```python
from build123d import *

# Parameters (mm, degrees)
SKETCH1_W                       = 90
SKETCH1_H                       = 40
BOSS_EXTRUDE1_DEPTH             = 20
SKETCH2_W                       = 20
SKETCH2_H                       = 10
CUT_EXTRUDE1_DEPTH              = 54.150729064
SKETCH3_W                       = 20
SKETCH3_H                       = 10
CUT_EXTRUDE2_DEPTH              = 54.150729064
SKETCH4_W                       = 20
SKETCH4_H                       = 10
CUT_EXTRUDE3_DEPTH              = 54.150729064
SKETCH5_W                       = 20
SKETCH5_H                       = 10
CUT_EXTRUDE4_DEPTH              = 54.150729064
F_5_0_5_DIAMETER_HOLE1_D        = 5
F_5_0_5_DIAMETER_HOLE1_DEPTH    = 12
M27_CLEARANCE_HOLE1_D           = 29.849192884
F_10_0_10_DIAMETER_HOLE1_REACH  = 63.033
F_10_0_10_DIAMETER_HOLE1_BORE_R = 5
F_12_0_12_DIAMETER_HOLE1_D      = 12
CHAMFER1_SIZE                   = 2
SKETCH18_R                      = 6.25
CUT_EXTRUDE6_DEPTH              = 100
SKETCH20_R                      = 15.175
CUT_EXTRUDE7_DEPTH              = 100
SKETCH21_R                      = 2.75
CUT_EXTRUDE8_DEPTH              = 12
SKETCH23_R                      = 5
BOSS_EXTRUDE2_DEPTH             = 20


with BuildPart() as part:
    # Sketch1 → Boss-Extrude1 (new body)
    with BuildSketch(Plane.XY.offset(10)):
        Rectangle(SKETCH1_W, SKETCH1_H)
    extrude(amount=-BOSS_EXTRUDE1_DEPTH)

    # Sketch2 → Cut-Extrude1 (cut, through all)
    with BuildSketch(Plane(origin=(0, 0, -10), x_dir=(-1, 0, 0), z_dir=(0, 0, -1))):
        with Locations((35, 15)):
            Rectangle(SKETCH2_W, SKETCH2_H)
    extrude(amount=-CUT_EXTRUDE1_DEPTH, mode=Mode.SUBTRACT)

    # Sketch3 → Cut-Extrude2 (cut, through all)
    with BuildSketch(Plane(origin=(0, 0, -10), x_dir=(-1, 0, 0), z_dir=(0, 0, -1))):
        with Locations((35, -15)):
            Rectangle(SKETCH3_W, SKETCH3_H)
    extrude(amount=-CUT_EXTRUDE2_DEPTH, mode=Mode.SUBTRACT)

    # Sketch4 → Cut-Extrude3 (cut, through all)
    with BuildSketch(Plane(origin=(0, 0, -10), x_dir=(-1, 0, 0), z_dir=(0, 0, -1))):
        with Locations((-35, -15)):
            Rectangle(SKETCH4_W, SKETCH4_H)
    extrude(amount=-CUT_EXTRUDE3_DEPTH, mode=Mode.SUBTRACT)

    # Sketch5 → Cut-Extrude4 (cut, through all)
    with BuildSketch(Plane(origin=(0, 0, -10), x_dir=(-1, 0, 0), z_dir=(0, 0, -1))):
        with Locations((-35, 15)):
            Rectangle(SKETCH5_W, SKETCH5_H)
    extrude(amount=-CUT_EXTRUDE4_DEPTH, mode=Mode.SUBTRACT)

    # Ø5.0 (5) Diameter Hole1
    with Locations(Plane.XY.offset(10)):
        with Locations((20, 0), (-20, 0)):
            Hole(F_5_0_5_DIAMETER_HOLE1_D / 2, depth=F_5_0_5_DIAMETER_HOLE1_DEPTH)

    # M27 Clearance Hole1 (through all)
    with Locations(Plane.XY.offset(10)):
        with Locations((0, 0)):
            Hole(M27_CLEARANCE_HOLE1_D / 2)

    # Ø10.0 (10) Diameter Hole1 bore → Ø10.0 (10) Diameter Hole1 (cut, up to next)
    with BuildSketch(Plane(origin=(0, -20, 0), x_dir=(-1, 0, 0), z_dir=(0, -1, 0)), mode=Mode.PRIVATE) as f_10_0_10_diameter_hole1_sk1:
        Circle(F_10_0_10_DIAMETER_HOLE1_BORE_R)
    f_10_0_10_diameter_hole1_tool1 = extrude(f_10_0_10_diameter_hole1_sk1.sketch, amount=-F_10_0_10_DIAMETER_HOLE1_REACH, mode=Mode.PRIVATE) & part.part
    add(f_10_0_10_diameter_hole1_tool1.solids().sort_by_distance((0, -20, 0))[0], mode=Mode.SUBTRACT)

    # Ø12.0 (12) Diameter Hole1 (through all)
    with Locations(Plane(origin=(0, 0, -10), x_dir=(-1, 0, 0), z_dir=(0, 0, -1))):
        with Locations((35, 0), (-35, 0)):
            Hole(F_12_0_12_DIAMETER_HOLE1_D / 2)

    # Chamfer1
    chamfer1_edges = [part.edges().sort_by_distance(p)[0] for p in [
        (-25, 20, 0),
        (-45, 10, 0),
        (-45, -10, 0),
        (-25, -20, 0),
        (25, -20, 0),
        (45, -10, 0),
        (45, 10, 0),
        (25, 20, 0),
    ]]
    chamfer(chamfer1_edges, length=CHAMFER1_SIZE)

    # Sketch18 → Cut-Extrude6 (cut)
    with BuildSketch(Plane.XY.offset(10)):
        with Locations((-35, 0)):
            Circle(SKETCH18_R)
        with Locations((35, 0)):
            Circle(SKETCH18_R)
    extrude(amount=-CUT_EXTRUDE6_DEPTH, mode=Mode.SUBTRACT)

    # Sketch20 → Cut-Extrude7 (cut)
    with BuildSketch(Plane.XY.offset(10)):
        Circle(SKETCH20_R)
    extrude(amount=-CUT_EXTRUDE7_DEPTH, mode=Mode.SUBTRACT)

    # Sketch21 → Cut-Extrude8 (cut)
    with BuildSketch(Plane.XY.offset(10)):
        with Locations((-20, 0)):
            Circle(SKETCH21_R)
        with Locations(Location((20, 0, 0), (0, 0, 180))):
            Circle(SKETCH21_R)
    extrude(amount=-CUT_EXTRUDE8_DEPTH, mode=Mode.SUBTRACT)

    # Sketch23 → Boss-Extrude2 (add)
    with BuildSketch(Plane.XZ.offset(10)):
        with Locations(Location((-33.846356211, 0, 0), (0, 0, 90))):
            Circle(SKETCH23_R)
        with Locations(Location((33.846356211, 0, 0), (0, 0, 90))):
            Circle(SKETCH23_R)
    extrude(amount=BOSS_EXTRUDE2_DEPTH)


solid = part.part
```
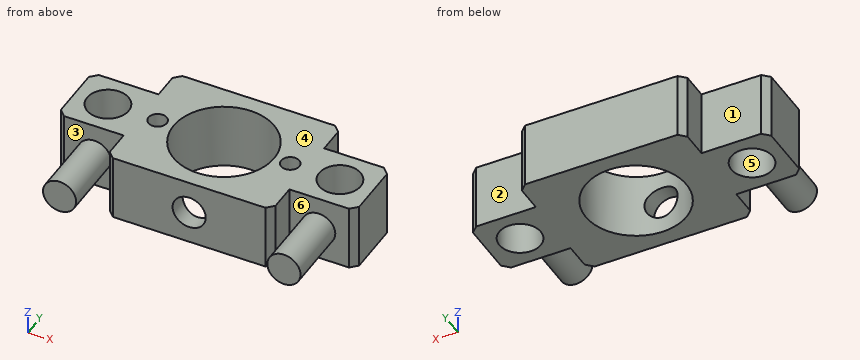
Verification items for the finished model (mm, model axes). Face numbers are marked on the shaded views. A direction names the side the tool comes from. Round coordinates to 2 decimals unless told otherwise and drop trailing zeros. Write each loop counter-clockwise with the first axis right and the second up, starting at its lowest first coordinate (ties: lowest second). Pieces come first, ordered by that corner, then holes.
1. Scan lines: L1, parallel to X at y = -16.55, z = 0; L2, parallel to X at y = -1, z = -1; L3, parallel to X at y = -16, z = -3.75. Record each from-to range of solid material in increasing order.
2. Section check B-B on x = 35. Enter the section's corners in (y, z), plus the area to 3 significant figures.
3. Access from +Z, -Z, +X, -X, +Y, -Y to the whole of each face (thin tool, end or side, straight path). Record for the marked faces 1, 2 and 3.
4. Draft check along Y on the marked faces 4, 5 and 6. Enter one of: +Y half, -Y half, draft (parallel to the pull), parting line (faces both ways), or undercut.
5. Section check D-D on z = 0. State how many separate pieces and enclosed holes the cut face has, plus the area to 3 significant figures.
6. Section check A-A on y = 0. Enter the section's corners in (x, z) (3 decimals).
7. Section check C-C on x = -2. Enter the section's corners in (y, z), plus the area to 3 significant figures.
8. Gauge pin test, flat ends, axial feed: P1, Ø2.5, axis at y = 12.5, z = 1, coming from the -X side; P2, Ø1.6, axis at x = 21, y = 1, coming from the +Z side; P3, Ø10, axis at x = -14.5, z = -4.5, coming from the -Y side. Record the tip position at first contact, or that the pin passes through.
Answer:
1. L1: x = -38.85 to -28.85, -25 to -5, 5 to 25, 28.85 to 38.85
1. L2: x = -45 to -41.17, -28.83 to -22.56, -17.44 to -15.14, 15.14 to 17.44, 22.56 to 28.83, 41.17 to 45
1. L3: x = -37.15 to -30.54, -25 to -3.31, 3.31 to 25, 30.54 to 37.15
2. outline: (-30, -4.87) - (-10, -4.87) - (-10, -10) - (-6.25, -10) - (-6.25, 10) - (-10, 10) - (-10, 4.87) - (-30, 4.87) - close; (6.25, -10) - (10, -10) - (10, 10) - (6.25, 10) - close
2. area: 345 mm2
3. face 1: +Z, -Z, -X, +Y
3. face 2: +Z, -Z, +X, +Y
3. face 3: -Y
4. face 4: draft
4. face 5: undercut
4. face 6: -Y half
5. separate pieces: 1
5. enclosed holes: 4
5. area: 2,120 mm2
6. outline: (-45, -10) - (-41.25, -10) - (-41.25, 10) - (-45, 10) - close; (-28.75, -10) - (-15.175, -10) - (-15.175, 10) - (-17.25, 10) - (-17.25, -2) - (-22.75, -2) - (-22.75, 10) - (-28.75, 10) - close; (15.175, -10) - (28.75, -10) - (28.75, 10) - (22.75, 10) - (22.75, -2) - (17.25, -2) - (17.25, 10) - (15.175, 10) - close; (41.25, -10) - (45, -10) - (45, 10) - (41.25, 10) - close
7. outline: (-20, -10) - (-15.04, -10) - (-15.04, -4.58) - (-20, -4.58) - close; (-20, 4.58) - (-15.04, 4.58) - (-15.04, 10) - (-20, 10) - close; (15.04, -10) - (20, -10) - (20, 10) - (15.04, 10) - close
7. area: 153 mm2
8. P1: stops at x = -25
8. P2: stops at z = -2
8. P3: stops at y = -20
